```python
from build123d import *

# Parameters (mm, degrees)
SKETCH_1_W          = 69
SKETCH_1_H          = 20
EXTRUDE_1_DEPTH     = 28
SKETCH_2_W          = 1.5
SKETCH_2_H          = 20
CUT_EXTRUDE_1_DEPTH = 22
SKETCH_3_R          = 1
CUT_EXTRUDE_2_DEPTH = 5
CUT_EXTRUDE_START   = -5
SKETCH_4_R          = 1
CUT_EXTRUDE_3_DEPTH = 5


with BuildPart() as part:
    # 草图1 → 拉伸1 (new body)
    with BuildSketch(Plane(origin=(0, 0, 0), x_dir=(1, 0, 0), z_dir=(0, 1, 0))):
        Rectangle(SKETCH_1_W, SKETCH_1_H)
    extrude(amount=EXTRUDE_1_DEPTH)

    # 草图2 → 切除-拉伸1 (cut)
    with BuildSketch(Plane(origin=(0, 28, 0), x_dir=(-1, 0, 0), z_dir=(0, 1, 0))):
        with Locations((-0.25, 0)):
            Rectangle(SKETCH_2_W, SKETCH_2_H)
        with Locations((2.25, 0)):
            Rectangle(SKETCH_2_W, SKETCH_2_H)
        with Locations((4.75, 0)):
            Rectangle(SKETCH_2_W, SKETCH_2_H)
        with Locations((7.25, 0)):
            Rectangle(SKETCH_2_W, SKETCH_2_H)
        with Locations((9.75, 0)):
            Rectangle(SKETCH_2_W, SKETCH_2_H)
        with Locations((12.25, 0)):
            Rectangle(SKETCH_2_W, SKETCH_2_H)
        with Locations((14.75, 0)):
            Rectangle(SKETCH_2_W, SKETCH_2_H)
        with Locations((17.25, 0)):
            Rectangle(SKETCH_2_W, SKETCH_2_H)
        with Locations((19.75, 0)):
            Rectangle(SKETCH_2_W, SKETCH_2_H)
        with Locations((22.25, 0)):
            Rectangle(SKETCH_2_W, SKETCH_2_H)
        with Locations((24.75, 0)):
            Rectangle(SKETCH_2_W, SKETCH_2_H)
        with Locations((27.25, 0)):
            Rectangle(SKETCH_2_W, SKETCH_2_H)
        with Locations((29.75, 0)):
            Rectangle(SKETCH_2_W, SKETCH_2_H)
        with Locations((32.25, 0)):
            Rectangle(SKETCH_2_W, SKETCH_2_H)
        with Locations((34.75, 0)):
            Rectangle(SKETCH_2_W, SKETCH_2_H)
        with Locations((-2.75, 0)):
            Rectangle(SKETCH_2_W, SKETCH_2_H)
        with Locations((-5.25, 0)):
            Rectangle(SKETCH_2_W, SKETCH_2_H)
        with Locations((-7.75, 0)):
            Rectangle(SKETCH_2_W, SKETCH_2_H)
        with Locations((-10.25, 0)):
            Rectangle(SKETCH_2_W, SKETCH_2_H)
        with Locations((-12.75, 0)):
            Rectangle(SKETCH_2_W, SKETCH_2_H)
        with Locations((-15.25, 0)):
            Rectangle(SKETCH_2_W, SKETCH_2_H)
        with Locations((-17.75, 0)):
            Rectangle(SKETCH_2_W, SKETCH_2_H)
        with Locations((-20.25, 0)):
            Rectangle(SKETCH_2_W, SKETCH_2_H)
        with Locations((-22.75, 0)):
            Rectangle(SKETCH_2_W, SKETCH_2_H)
        with Locations((-25.25, 0)):
            Rectangle(SKETCH_2_W, SKETCH_2_H)
        with Locations((-27.75, 0)):
            Rectangle(SKETCH_2_W, SKETCH_2_H)
        with Locations((-30.25, 0)):
            Rectangle(SKETCH_2_W, SKETCH_2_H)
        with Locations((-32.75, 0)):
            Rectangle(SKETCH_2_W, SKETCH_2_H)
    extrude(amount=-CUT_EXTRUDE_1_DEPTH, mode=Mode.SUBTRACT)

    # 草图3 → 切除-拉伸2 (cut)
    with BuildSketch(Plane.ZY.offset(34)):
        with Locations((0, 8)):
            Circle(SKETCH_3_R)
    extrude(amount=-CUT_EXTRUDE_2_DEPTH, mode=Mode.SUBTRACT)

    # 草图4 → 切除-拉伸3 (cut)
    with BuildSketch(Plane(origin=(34.5, 0, 0), x_dir=(0, 0, -1), z_dir=(1, 0, 0)).offset(CUT_EXTRUDE_START)):
        with Locations(Location((0, 8, 0), (0, 0, 180))):
            Circle(SKETCH_4_R)
    extrude(amount=CUT_EXTRUDE_3_DEPTH, mode=Mode.SUBTRACT)


solid = part.part
```
Can you work these out from the model? Positions are in its coordinate system, mm. A direction names the side the tool comes from. Coordinates: 2 decimals unless noted, no trailing zeros.
1. Thinking about a two-plate mould opening in X: for faces 1 (the face through (34, 7, 0)), 2 (the face through (-34.5, 3, 0)), 3 (the face through (14.5, 17, 0)), 4 (the face through (-30, 6, 0)), which applies, +X half, -X half, draft (parallel to the pull), parting line (faces both ways), or undercut?
2. If we section it at A-A (z = 0): Give the number of separate pieces and of enclosed holes in the cut face, then the cut area to 3 significant figures.
3. I need wall thicknesses on line 1 (Z direction, x = 34, y = 8); line 2 (Y direction, x = -33.6, z = 0); line 3 (Y direction, x = -20, z = -6.25). Which ranges of each line are inside material? Lowest first, please.
4. I'm going to push flat-ended pins straight in: pin 1 (0.8 mm diameter, centred on x = -4.5, z = -2, fed in from +Y); pin 2 (6 mm diameter, centred on y = 21.5, z = 4.5, fed in from -X). Where does each tip first touch, or does it pass through?
5. For faces 5 (the face through (-20.5, 17, 0)), 6 (the face through (31.49, 7.01, -0.13)), which set-ups out of +Z, -Z, +X, -X, +Y, -Y let a thin tool reach every point of the face, with its end or its side?
Entries:
1. face 1: draft
1. face 2: -X half
1. face 3: undercut
1. face 4: undercut
2. separate pieces: 5
2. enclosed holes: 0
2. area: 1,020 mm2
3. line 1: z = -10 to -1, 1 to 10
3. line 2: y = 0 to 7, 9 to 28
3. line 3: y = 0 to 6
4. pin 1: stops at y = 6
4. pin 2: stops at x = -34
5. face 5: +Z, -Z, +Y
5. face 6: +X
